from build123d import *

# Parameters (mm, degrees)
SKETCH1_W           = 4.7625
SKETCH1_H           = 4.7625
SKETCH1_W_2         = 3.96875
SKETCH1_H_2         = 3.96875
BOSS_EXTRUDE1_DEPTH = 15
SKETCH2_R           = 0.79375
CUT_EXTRUDE1_DEPTH  = 16.917027292


with BuildPart() as part:
    # Sketch1 → Boss-Extrude1 (new, symmetric)
    with BuildSketch(Plane.XY):
        Rectangle(SKETCH1_W, SKETCH1_H)
        Rectangle(SKETCH1_W_2, SKETCH1_H_2, mode=Mode.SUBTRACT)
    extrude(amount=BOSS_EXTRUDE1_DEPTH, both=True)

    # Sketch2 → Cut-Extrude1 (cut, through all)
    with BuildSketch(Plane.ZY.offset(2.38125)):
        with Locations((-11, 0)):
            Circle(SKETCH2_R)
        with Locations((11, 0)):
            Circle(SKETCH2_R)
    extrude(amount=-CUT_EXTRUDE1_DEPTH, mode=Mode.SUBTRACT)


solid = part.part
CAD build for the part. Positions are in the model's coordinates, mm. A direction names the side the tool comes from. Give positions to 0.01 mm unless a question says otherwise; leave off trailing zeros. Write each loop counter-clockwise with the first axis right and the second up, starting at its lowest first coordinate (ties: lowest second). Pieces come first, ordered by that corner, then holes. Notation, with made-up numbers: M -4.5,21.5 L 27.5,21.5 A28 ccw 27.5,48.5 Z; hole C 57,-21.75 d8. An arc over 180 degrees is marked long. Put each result on its own line as item: value. Start each with the question number.
(1) Band-saw the part on C-C, the plane y = 0. Write the cut outline in (x, z), and give its area (3 significant figures).
(2) Flat gauge pin, fed straight in: pin 1 Ø1.3 at (y, z) = (0, 11) entering from +X. Where does the tip first touch, or does it go through?
(3) Which spindle directions (+Z, -Z, +X, -X, +Y, -Y) get a long thin tool onto all of the face, cutting with end or side? Do faces 1 (the face through (-2.2, 0, 15)), 2 (the face through (0, 1.984, 0)). Say none if no direction does.
(4) Band-saw the part on B-B, the plane x = 0.8. Write the cut outline in (y, z).
(5) Probe L1, parallel to X at y = 1.05, z = 13; L2, parallel to Y at x = 2.3, z = -11. List the from-to ranges inside material, lowest first.
(6) Mould opens along Z. For faces 3 (the face through (2.18, 0.238, 11.757)), 4 (the face through (-2.2, 0, -15)), 5 (the face through (2.381, 0, 0)) say: +Z half, -Z half, draft (parallel to the pull), parting line (faces both ways), or undercut.
(7) Band-saw the part on D-D, the plane z = -0.75. Write the cut outline in (x, y).
(8) Band-saw the part on A-A, the plane z = -11. Write the cut outline in (x, y), and give its area (3 significant figures).
Response values:
1. outline: M -2.38,-15 L -1.98,-15 L -1.98,-11.79 L -2.38,-11.79 Z; M -2.38,-10.21 L -1.98,-10.21 L -1.98,10.21 L -2.38,10.21 Z; M -2.38,11.79 L -1.98,11.79 L -1.98,15 L -2.38,15 Z; M 1.98,-15 L 2.38,-15 L 2.38,-11.79 L 1.98,-11.79 Z; M 1.98,-10.21 L 2.38,-10.21 L 2.38,10.21 L 1.98,10.21 Z; M 1.98,11.79 L 2.38,11.79 L 2.38,15 L 1.98,15 Z
1. area: 21.3 mm2
2. pin 1: passes through
3. face 1: +Z, +X, -X, +Y, -Y
3. face 2: +Z, -Z
4. outline: M -2.38,-15 L -1.98,-15 L -1.98,15 L -2.38,15 Z; M 1.98,-15 L 2.38,-15 L 2.38,15 L 1.98,15 Z
5. L1: x = -2.38 to -1.98, 1.98 to 2.38
5. L2: y = -2.38 to -0.79, 0.79 to 2.38
6. face 3: undercut
6. face 4: -Z half
6. face 5: draft
7. outline: M -2.38,-2.38 L 2.38,-2.38 L 2.38,2.38 L -2.38,2.38 Z; hole M -1.98,-1.98 L 1.98,-1.98 L 1.98,1.98 L -1.98,1.98 Z
8. outline: M -2.38,-2.38 L 2.38,-2.38 L 2.38,-0.79 L 1.98,-0.79 L 1.98,-1.98 L -1.98,-1.98 L -1.98,-0.79 L -2.38,-0.79 Z; M -2.38,0.79 L -1.98,0.79 L -1.98,1.98 L 1.98,1.98 L 1.98,0.79 L 2.38,0.79 L 2.38,2.38 L -2.38,2.38 Z
8. area: 5.67 mm2
